Can you work these out from the model? Positions are in its coordinate system, mm. A direction names the side the tool comes from. Coordinates: 2 decimals unless noted, no trailing zeros. Loops run counter-clockwise (first coordinate to the right, second up) from the corner with the lowest first, then second, coordinate; pieces in that order, holes last. Notation, with made-up numbers: (-36.75, 38.25) - (-22.75, 38.25) arc R33 ccw to (-22.75, 75.25) - close; hole circle Ø10 at (-3, 12). An arc over 180 degrees is marked (long way). Put each result on its own line as item: value. Start each with the question number.
from build123d import *

# Parameters (mm, degrees)
SKETCH2_W           = 24
SKETCH2_H           = 24
BOSS_EXTRUDE1_DEPTH = 77
SKETCH3_W           = 3.6
SKETCH3_H           = 12
CUT_EXTRUDE3_DEPTH  = 77
SKETCH4_R           = 2.1
SKETCH4_R_2         = 4.5
CUT_EXTRUDE4_DEPTH  = 8.4


with BuildPart() as part:
    # Sketch2 → Boss-Extrude1 (new body)
    with BuildSketch(Plane(origin=(0, 0, 0), x_dir=(0, 0, -1), z_dir=(1, 0, 0))):
        Rectangle(SKETCH2_W, SKETCH2_H)
    extrude(amount=BOSS_EXTRUDE1_DEPTH)

    # Sketch3 → Cut-Extrude3 (cut)
    with BuildSketch(Plane(origin=(77, 0, 0), x_dir=(0, 0, -1), z_dir=(1, 0, 0))):
        with Locations((1.8, -6)):
            Rectangle(SKETCH3_W, SKETCH3_H)
    cut_extrude3 = extrude(amount=-CUT_EXTRUDE3_DEPTH, mode=Mode.SUBTRACT)

    # Mirror1: Cut-Extrude3 across plane
    add(cut_extrude3.mirror(Plane.XY), mode=Mode.SUBTRACT)

    # Sketch4 → Cut-Extrude4 (cut)
    with BuildSketch(Plane.XY.offset(-12)):
        with Locations(Location((40, 2, 0), (0, 0, 252.247209838))):
            Circle(SKETCH4_R)
        with Locations(Location((22.5, -6, 0), (0, 0, 90))):
            Circle(SKETCH4_R_2)
        with Locations(Location((5, 2, 0), (0, 0, 252.247209838))):
            Circle(SKETCH4_R)
    extrude(amount=CUT_EXTRUDE4_DEPTH, mode=Mode.SUBTRACT)


solid = part.part
Q1. On a 3-axis mill with a long thin cutter (end or side, diameter ignored), from which of +Z, -Z, +X, -X, +Y, -Y can I reach the whole of each face in a straight line? I mean faces 4 (the flat face through (38, -12, -8)), 5 (the cylindrical face through (7.066, 1.625, -7.859)), 6 (the flat face through (39, -6, 3.6)). Say none if no direction works.
Q2. I want a section at D-D on z = -2.75. List the corners of the cut face in (x, y) for me, and give its area (3 significant figures).
Q3. Please list where these lines run through material, in increasing order: line 1 along X through (y, z) = (2, -8.75); line 2 along Z through (x, y) = (61.5, -2); line 3 along Y through (x, z) = (5, -9.5). Write a range as [from, to].
Q4. I want a section at B-B on x = 29. List the corners of the cut face in (y, z) for me.
Q5. I want a section at A-A on y = -5.5. List the corners of the cut face in (x, z) for me.
Q6. I want a section at C-C on y = 2. List the corners of the cut face in (x, z) for me.
Q7. Will these pins go through, and if not, where does the flat tip stop? pin 1 (1.2 mm diameter, centred on x = 5, y = 1, fed in from -Z); pin 2 (5.5 mm diameter, centred on x = 22.5, y = -6, fed in from -Z); pin 3 (3 mm diameter, centred on x = 28.5, z = -1, fed in from -Y).
Q8. We'd pull the mould along Z, two halves only. Please class faces 1 (the flat face through (38, 12, 0)), 2 (the flat face through (39, -6, -3.6)), 3 (the flat face through (5, 2, -3.6)): released by +Z, released by -Z, zero draft, split by the parting line, or undercut.
Calculated:
1. face 4: +Z, -Z, +X, -X, -Y
1. face 5: -Z
1. face 6: +X, -X, -Y
2. outline: (0, 0) - (77, 0) - (77, 12) - (0, 12) - close
2. area: 924 mm2
3. line 1: [0, 2.9], [7.1, 37.9], [42.1, 77]
3. line 2: [-12, -3.6], [3.6, 12]
3. line 3: [-12, -0.1], [4.1, 12]
4. outline: (-12, -12) - (12, -12) - (12, 12) - (-12, 12) - (-12, 3.6) - (0, 3.6) - (0, -3.6) - (-12, -3.6) - close
5. outline: (0, -12) - (18.03, -12) - (18.03, -3.6) - (0, -3.6) - close; (0, 3.6) - (77, 3.6) - (77, 12) - (0, 12) - close; (26.97, -12) - (77, -12) - (77, -3.6) - (26.97, -3.6) - close
6. outline: (0, -12) - (2.9, -12) - (2.9, -3.6) - (7.1, -3.6) - (7.1, -12) - (37.9, -12) - (37.9, -3.6) - (42.1, -3.6) - (42.1, -12) - (77, -12) - (77, 12) - (0, 12) - close
7. pin 1: z = -3.6
7. pin 2: z = 3.6
7. pin 3: y = 0
8. face 1: zero draft
8. face 2: undercut
8. face 3: released by -Z
